Geometry check sheet. Reference: the model listing, model coordinates, mm. Coordinates: 2 decimals unless noted, no trailing zeros. Write each loop counter-clockwise with the first axis right and the second up, starting at its lowest first coordinate (ties: lowest second). Pieces come first, ordered by that corner, then holes. Notation, with made-up numbers: (58.25, -25.75) -> (77.25, -25.75) arc R14 ccw to (77.25, -2.75) -> close; hole circle Ø11 at (37.5, -11.5). An arc over 180 degrees is marked (long way). Use a Markdown table: item, result.
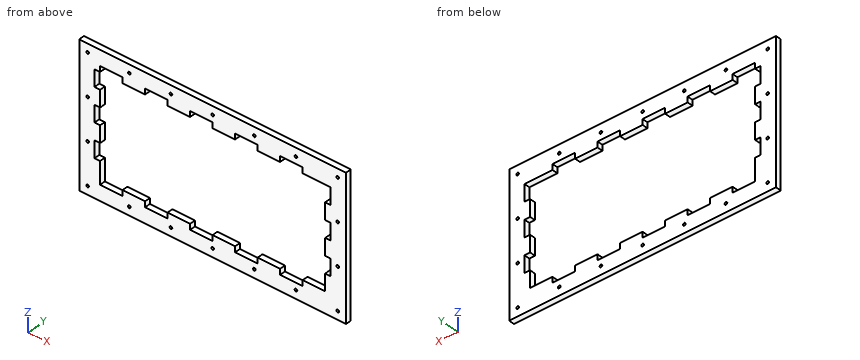
Autodesk Inventor part; units mm, degrees
ref_plane "YZ Plane" through (0, 0, 0) normal (1, 0, 0) x (0, 1, 0)
ref_plane "XZ Plane" through (0, 0, 0) normal (0, 1, 0) x (-1, 0, 0)
ref_plane "XY Plane" through (0, 0, 0) normal (0, 0, 1) x (1, 0, 0)
sketch "Sketch1" plane through (0, 0, 0) normal (0, 1, 0) x (-1, 0, 0)
  line L0 (0, 0) -> (320, 0)
  line L1 (320, 0) -> (320, -170)
  line L2 (320, -170) -> (0, -170)
  line L3 (0, -170) -> (0, 0)
  line L4 (0, 0) -> (25, 0)
  line L5 (25, -25) -> (295, -25)
  line L6 (295, -25) -> (295, -145)
  line L7 (295, -145) -> (25, -145)
  line L8 (25, -145) -> (25, -25)
  dimension "d0" = 320
  dimension "d1" = 170
  dimension "d2" = 25
  dimension "d3" = 25
  dimension "d4" = 270
  dimension "d5" = 120
extrude "Extrusion1" add sketch "Sketch1" along normal blind 6.7
sketch "Sketch2" plane through (0, 6.7, 0) normal (0, 1, 0) x (1, 0, 0)
  line L0 (-320, 0) -> (0, 0)
  line L1 (0, 0) -> (0, 170)
  circle A0 centre (-10, 10) radius 1.6
  line L2 (0, 170) -> (0, 160)
  circle A1 centre (-10, 160) radius 1.6
  dimension "d10" = 3.2
  dimension "d13" = 3.2
extrude "Extrusion2" cut sketch "Sketch2" against normal blind 6.7
pattern_linear "Rectangular Pattern1" count 7 spacing 50 along (-1, 0, 0) of "Extrusion2"
sketch "Sketch3" plane through (0, 6.7, 0) normal (0, 1, 0) x (1, 0, 0)
  circle A0 centre (-310, 10) radius 1.6
  circle A1 centre (-310, 60) radius 1.6
  circle A2 centre (-10, 10) radius 1.6
  circle A3 centre (-10, 60) radius 1.6
  point P0 (0, 0)
  dimension "d20" = 3.2
  dimension "d22" = 3.2
extrude "Extrusion3" cut sketch "Sketch3" against normal blind 6.7 contours A1 | A3
pattern_linear "Rectangular Pattern2" count 2 spacing 50 along (0, 0, -1) of "Extrusion3"
sketch "Sketch4" plane through (0, 6.7, 0) normal (0, 1, 0) x (1, 0, 0)
  line L0 (-25, 25) -> (-25, 145)
  line L1 (-25, 25) -> (-295, 25)
  line L2 (-52, 25) -> (-79, 25)
  line L3 (-79, 25) -> (-79, 18.3)
  line L4 (-79, 18.3) -> (-52, 18.3)
  line L5 (-52, 18.3) -> (-52, 25)
  line L6 (-295, 145) -> (-25, 145)
  line L7 (-25, 145) -> (-52, 145)
  line L8 (-52, 145) -> (-79, 145)
  line L9 (-79, 145) -> (-79, 151.7)
  line L10 (-79, 151.7) -> (-52, 151.7)
  line L11 (-52, 151.7) -> (-52, 145)
  point P0 (0, 0)
  dimension "d28" = 27
  dimension "d29" = 27
  dimension "d30" = 6.7
  dimension "d31" = 27
  dimension "d32" = 27
  dimension "d33" = 6.7
extrude "Extrusion4" cut sketch "Sketch4" against normal blind 6.7
pattern_linear "Rectangular Pattern3" count 5 spacing 54 along (-1, 0, 0) of "Extrusion4"
sketch "Sketch5" plane through (0, 6.7, 0) normal (0, 1, 0) x (1, 0, 0)
  line L0 (-25, 145) -> (-25, 25)
  line L1 (-25, 25) -> (-18.3, 25)
  line L2 (-18.3, 25) -> (-18.3, 45)
  line L3 (-18.3, 45) -> (-25, 45)
  line L4 (-25, 45) -> (-25, 25)
  line L5 (-295, 18.3) -> (-295, 151.7)
  line L6 (-295, 25) -> (-301.7, 25)
  line L7 (-301.7, 25) -> (-301.7, 45)
  line L8 (-301.7, 45) -> (-295, 45)
  line L9 (-295, 45) -> (-295, 25)
  point P0 (0, 0)
  dimension "d39" = 6.7
  dimension "d40" = 20
  dimension "d41" = 6.7
  dimension "d42" = 20
extrude "Extrusion5" cut sketch "Sketch5" against normal blind 6.7
pattern_linear "Rectangular Pattern4" count 3 spacing 40 along (0, 0, -1) of "Extrusion5"
properties part number "b_Base_support 1"
Item 1: Section check B-B on x = -195.5. Record the boundary of the cut face in (y, z).
Answer block:
| item | result |
|---|---|
| outline | (0, -170) -> (6.7, -170) -> (6.7, -145) -> (0, -145) -> close; (0, -25) -> (6.7, -25) -> (6.7, 0) -> (0, 0) -> close |
Item 2: Section check C-C on y = 4.5. Count the separate pieces of the cut face and the enclosed holes in it, then the cut area to 3 significant figures.
Answer block:
| item | result |
|---|---|
| separate pieces | 1 |
| enclosed holes | 19 |
| area | 19,200 mm^2 |
Item 3: Section check A-A on z = -95. Record the boundary of the cut face in (x, y).
Answer block:
| item | result |
|---|---|
| outline | (-320, 0) -> (-295, 0) -> (-295, 6.7) -> (-320, 6.7) -> close; (-25, 0) -> (0, 0) -> (0, 6.7) -> (-25, 6.7) -> close |
Item 4: Thickness scan on L1, parallel to Z at x = -210, y = 3.75; L2, parallel to X at y = 2.5, z = -110; L3, parallel to Z at x = -310, y = 5. Record the ranges inside material, lowest first. Write a range as [from, to].
Answer block:
| item | result |
|---|---|
| L1 | z = [-170, -161.6], [-158.4, -145], [-25, -11.6], [-8.4, 0] |
| L2 | x = [-320, -311.6], [-308.4, -301.7], [-18.3, -11.6], [-8.4, 0] |
| L3 | z = [-170, -161.6], [-158.4, -111.6], [-108.4, -61.6], [-58.4, -11.6], [-8.4, 0] |
